Read the model definition and answer for the solid it produces. Units are mm, in the model's axes. Face numbers are marked on the shaded views. Coordinates: 2 decimals unless noted, no trailing zeros. Write each loop counter-clockwise with the first axis right and the second up, starting at its lowest first coordinate (ties: lowest second). Pieces come first, ordered by that corner, then holes. Notation, with made-up numbers: M 9.25,13.5 L 25.25,13.5 A13 cw 25.25,19.5 Z; hole C 39.25,82 d5. An arc over 180 degrees is marked long. Write item = value, one per line.
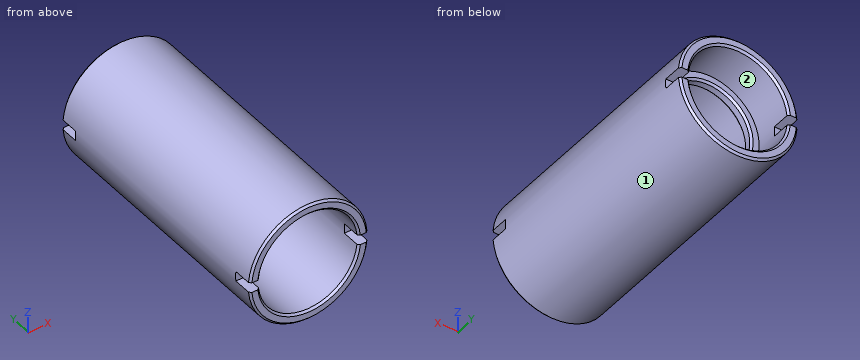
from build123d import *

# Parameters (mm, degrees)
SKETCH2_W          = 70
SKETCH2_H          = 5
CUT_EXTRUDE1_DEPTH = 10
SKETCH3_W          = 70
SKETCH3_H          = 5
CUT_EXTRUDE2_DEPTH = 10
CHAMFER1_SIZE      = 1


with BuildPart() as part:
    # Sketch1 → Revolve1 (revolve)
    with BuildSketch(Plane.XY):
        Polygon((25, -134), (30, -134), (30, 0), (25, 0), (25, -21), (21, -21), (21, -26), (25, -26), align=None)
    revolve(axis=Axis((0, 0, 0), (0, 1, 0)))

    # Sketch2 → Cut-Extrude1 (cut)
    with BuildSketch(Plane(origin=(0, 0, 0), x_dir=(1, 0, 0), z_dir=(0, 1, 0))):
        Rectangle(SKETCH2_W, SKETCH2_H)
    extrude(amount=-CUT_EXTRUDE1_DEPTH, mode=Mode.SUBTRACT)

    # Sketch3 → Cut-Extrude2 (cut)
    with BuildSketch(Plane.XZ.offset(134)):
        Rectangle(SKETCH3_W, SKETCH3_H)
    extrude(amount=-CUT_EXTRUDE2_DEPTH, mode=Mode.SUBTRACT)

    # Chamfer1
    chamfer1_edges = [part.edges().sort_by_distance(p)[0] for p in [
        (-21, -26, 0),
        (-21, -21, 0),
        (0, 0, 25),
        (0, 0, -25),
        (0, 0, 30),
        (0, 0, -30),
        (0, -134, 30),
        (0, -134, -30),
        (0, -134, 25),
        (0, -134, -25),
    ]]
    chamfer(chamfer1_edges, length=CHAMFER1_SIZE)


solid = part.part
Item 1: Flat-ended cylindrical pins translate along their axes: pin 1 (4 mm diameter, centred on x = 28, y = -131, fed in from -Z); pin 2 (5.5 mm diameter, centred on x = 28, y = -2.5, fed in from +Z); pin 3 (3 mm diameter, centred on x = 21.5, y = -42, fed in from +Z); pin 4 (12 mm diameter, centred on x = 15.5, z = 16, fed in from -Y). Find the tip coordinate at first contact, or state that the pin passes through.
Worked answers:
pin_1 = -14.97
pin_2 = 16.2
pin_3 = 22.36
pin_4 = -134
Item 2: Consider line 1 along X through (y, z) = (-23, 0); line 2 along Y through (x, z) = (1.5, 22.5); line 3 along Z through (x, y) = (1, -118.5). Determine where each line is inside the solid, lowest interval first. Write a range as from..to.
Worked answers:
line_1 = -30..-21, 21..30
line_2 = -26..-21
line_3 = -29.98..-24.98, 24.98..29.98
Item 3: Find section A-A (z = 0). Determine the outline of the cut face in (x, y).
Worked answers:
outline = M -30,-124 L -25,-124 L -25,-26 L -22,-26 L -21,-25 L -21,-22 L -22,-21 L -25,-21 L -25,-10 L -30,-10 Z; M 21,-25 L 22,-26 L 25,-26 L 25,-124 L 30,-124 L 30,-10 L 25,-10 L 25,-21 L 22,-21 L 21,-22 Z
Item 4: Find section C-C (y = -46). Determine the outline of the cut face in (x, z), and give its area (3 significant figures).
Worked answers:
outline = C 0,0 d60; hole C 0,0 d50
area = 864 mm²
Item 5: Find section B-B (x = 0). Determine the outline of the cut face in (y, z).
Worked answers:
outline = M -134,-29 L -133,-30 L -1,-30 L 0,-29 L 0,-26 L -1,-25 L -21,-25 L -21,-22 L -22,-21 L -25,-21 L -26,-22 L -26,-25 L -133,-25 L -134,-26 Z; M -134,26 L -133,25 L -26,25 L -26,22 L -25,21 L -22,21 L -21,22 L -21,25 L -1,25 L 0,26 L 0,29 L -1,30 L -133,30 L -134,29 Z
Item 6: For a pull along X with two mould halves and no side action, classify the marked faces 1 and 2 as released by +X, released by -X, zero draft, split by the parting line, or undercut.
Worked answers:
face_1 = split by the parting line
face_2 = undercut
